For this review, take the finished solid that the model builds, in its own axes (mm). Face numbers are marked on the shaded views. A direction names the side the tool comes from. Coordinates: 2 decimals unless noted, no trailing zeros. Loops run counter-clockwise (first coordinate to the right, second up) from the corner with the lowest first, then second, coordinate; pieces in that order, holes last. Notation, with made-up numbers: M 78,-6.5 L 82,-6.5 A26 ccw 82,27.5 Z; hole C 68,59.25 d4. An arc over 180 degrees is marked long. Answer as a JSON object with one key per item and string values. Group by question number.
Item 1: Mouldability with a two-part tool opening along X and no side actions: class the marked faces 3, 4, 5 and 6 as +X half, -X half, draft (parallel to the pull), parting line (faces both ways), or undercut.
Item 2: Add section D-D (x = 1.5). State the section outline as (y, z) points, then the cut area to 3 significant figures.
Item 3: Add section C-C (z = 5). State the section outline as (x, y) points, then the cut area to 3 significant figures.
Item 4: Add section B-B (y = 7.25). State the section outline as (x, z) points, then the cut area to 3 significant figures.
Item 5: Insertion check: pin 1 (2 mm diameter, centred on y = 3, z = -1.5, fed in from -X); pin 2 (3 mm diameter, centred on x = 1.5, z = -0.5, fed in from +Y); pin 3 (4 mm diameter, centred on y = 11, z = -0.5, fed in from +X). Each pin has a flat end and moves straight along its axis. Give the tip position at first contact, or say it passes through.
Item 6: Wall thickness on L1, parallel to X at y = 8.25, z = 0; L2, parallel to Y at x = 2.75, z = -5; L3, parallel to X at y = 10.75, z = 1.25: over which ranges is each line inside the solid? List them lowest first. Write a range as from..to.
Item 7: Tool access review of the marked faces 1 and 2: name each direction out of +Z, -Z, +X, -X, +Y, -Y from which nothing blocks a thin tool from reaching the whole face with its end or side.
Item 8: Add section A-A (x = 0). State the section outline as (y, z) points, then the cut area to 3 significant figures.
from build123d import *

# Parameters (mm, degrees)
SKETCH_1_R          = 2
EXTRUDE_1_DEPTH     = 18
SKETCH_2_R          = 5.5
SKETCH_2_R_2        = 3.5
CUT_EXTRUDE_2_DEPTH = 13.5


with BuildPart() as part:
    # 草图1 → 凸台-拉伸1 (new body)
    with BuildSketch(Plane(origin=(0, 0, 0), x_dir=(1, 0, 0), z_dir=(0, 1, 0))):
        Polygon((6.92820323, 0), (3.464101615, 6), (-3.464101615, 6), (-6.92820323, 0), (-3.464101615, -6), (3.464101615, -6), align=None)
        with Locations(Location((0, 0, 0), (0, 0, 270))):
            Circle(SKETCH_1_R, mode=Mode.SUBTRACT)
    extrude(amount=EXTRUDE_1_DEPTH)

    # 草图2 → 切除-拉伸2 (cut)
    # profile 1 of 2: a face of its own
    with BuildSketch(Plane(origin=(0, 18, 0), x_dir=(1, 0, 0), z_dir=(0, 1, 0))):
        Polygon((-6.92820323, 0), (-3.464101615, -6), (3.464101615, -6), (6.92820323, 0), (3.464101615, 6), (-3.464101615, 6), align=None)
        with Locations(Location((0, 0, 0), (0, 0, 270))):
            Circle(SKETCH_2_R, mode=Mode.SUBTRACT)
    # profile 2 of 2: a face of its own
    with BuildSketch(Plane(origin=(0, 18, 0), x_dir=(1, 0, 0), z_dir=(0, 1, 0))):
        with Locations(Location((0, 0, 0), (0, 0, 270))):
            Circle(SKETCH_2_R_2)
    extrude(amount=-CUT_EXTRUDE_2_DEPTH, mode=Mode.SUBTRACT)


solid = part.part
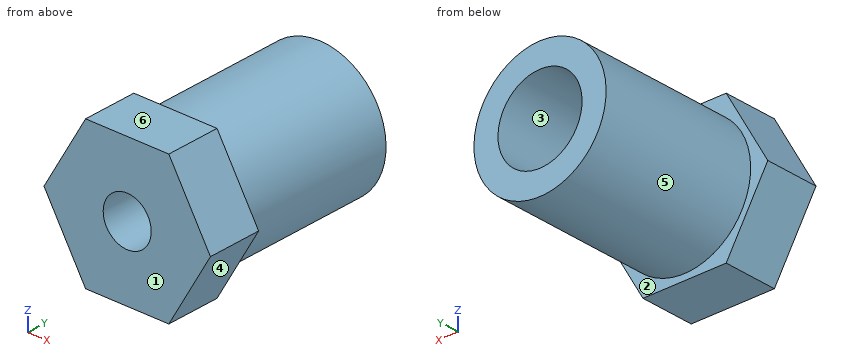
From the geometry:
{
 "1": {"face 3": "undercut", "face 4": "+X half", "face 5": "parting line", "face 6": "draft"},
 "2": {"outline": "M 0,-6 L 4.5,-6 L 4.5,-5.29 L 18,-5.29 L 18,-3.16 L 4.5,-3.16 L 4.5,-1.32 L 0,-1.32 Z; M 0,1.32 L 4.5,1.32 L 4.5,3.16 L 18,3.16 L 18,5.29 L 4.5,5.29 L 4.5,6 L 0,6 Z", "area": "99.6 mm²"},
 "3": {"outline": "M -4.04,0 L 4.04,0 L 4.04,4.5 L 2.29,4.5 L 2.29,18 L -2.29,18 L -2.29,4.5 L -4.04,4.5 Z", "area": "98.2 mm²"},
 "4": {"outline": "C 0,0 d11; hole C 0,0 d7", "area": "56.5 mm²"},
 "5": {"pin 1": "stops at x = -6.64", "pin 2": "stops at y = 4.5", "pin 3": "stops at x = 5.5"},
 "6": {"L1": "x = -5.5..-3.5, 3.5..5.5", "L2": "y = 0..4.5", "L3": "x = -5.36..-3.27, 3.27..5.36"},
 "7": {"face 1": "+Z, -Z, +X, -X, -Y", "face 2": "+Y"},
 "8": {"outline": "M 0,-6 L 4.5,-6 L 4.5,-5.5 L 18,-5.5 L 18,-3.5 L 4.5,-3.5 L 4.5,-2 L 0,-2 Z; M 0,2 L 4.5,2 L 4.5,3.5 L 18,3.5 L 18,5.5 L 4.5,5.5 L 4.5,6 L 0,6 Z", "area": "90.0 mm²"}
}
